Read the model definition and answer for the solid it produces. Units are mm, in the model's axes. Face numbers are marked on the shaded views. A direction names the side the tool comes from. Give positions to 0.01 mm unless a question says otherwise; leave off trailing zeros. Order: outer loops, then holes, each group sorted by start corner. A loop starts at its lowest first (then second) coordinate and runs counter-clockwise, first axis right, second up. Notation, with made-up numbers: (48, 70) - (70, 70) arc R20 cw to (70, 77) - close; hole circle Ø6 at (85.5, 44.25). An arc over 180 degrees is marked (long way). Use a Markdown table: item, result. Add a question column.
1. Which of the six approach directions +Z, -Z, +X, -X, +Y, -Y give full straight-line access (tool end or side, diameter ignored) to the marked faces 4, 5 and 6?
2. A cutting plane is placed at A-A on z = -11. Determine the outline of the cut face in (x, y) (1 decimal).
3. For a pull along X with two mould halves and no side action, classify the marked faces 1, 2 and 3 as released by +X, released by -X, zero draft, split by the parting line, or undercut.
4. Flat-ended cylindrical pins translate along their axes: P1, Ø3, axis at x = 14, z = -22.5, coming from the +Y side; P2, Ø1, axis at x = 20, z = -21, coming from the +Y side; P3, Ø6, axis at x = 3.5, z = -13, coming from the +Y side; P4, Ø3.5, axis at y = 0, z = 0, coming from the +X side. Find the tip coordinate at first contact, or state that the pin passes through.
5. A cutting plane is placed at D-D on x = 16.25. Determine the outline of the cut face in (y, z), and give its area (3 significant figures).
6. Consider L1, parallel to X at y = 1, z = -9 (1 decimal); L2, parallel to Y at x = 26, z = -14.5; L3, parallel to Z at x = 2.5, y = 0. Determine where each line is inside the solid, lowest interval first.
7. A cutting plane is placed at B-B on x = 22.25. Determine the outline of the cut face in (y, z) (1 decimal), and give its area (3 significant figures).
8. A cutting plane is placed at C-C on z = -1.5. Determine the outline of the cut face in (x, y) (1 decimal), and give its area (3 significant figures).
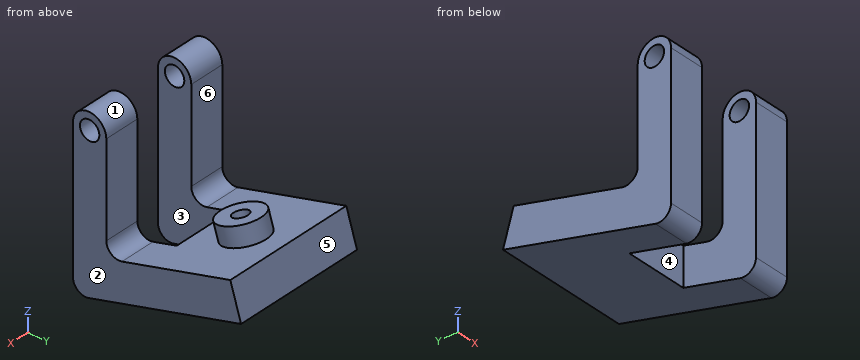
```python
from build123d import *

# Parameters (mm, degrees)
SKETCH1_R               = 2.032
BOSS_EXTRUDE1_DEPTH     = 27.305
FILLET1_R               = 2.54
SKETCH2_W               = 12.7
SKETCH2_H               = 15.24
CUT_EXTRUDE1_DEPTH      = 4.4925
CUT_EXTRUDE1_DEPTH_BACK = 33.127387008
SKETCH3_R               = 4.445
SKETCH3_R_2             = 1.5875
BOSS_EXTRUDE2_DEPTH     = 3.796503


with BuildPart() as part:
    # Sketch1 → Boss-Extrude1 (new body)
    with BuildSketch(Plane(origin=(0, 0, 0), x_dir=(0, 0, -1), z_dir=(1, 0, 0))):
        with BuildLine():
            Line((0, 3.4925), (22.86, 3.4925))
            Line((22.86, 3.4925), (14.913420462, 29.48459049))
            Line((14.913420462, 29.48459049), (22.251950115, 31.728204162))
            Line((22.251950115, 31.728204162), (33.02, -3.4925))
            Line((33.02, -3.4925), (0, -3.4925))
            ThreePointArc((0, -3.4925), (-3.4925, 0), (0, 3.4925))
        make_face()
        Circle(SKETCH1_R, mode=Mode.SUBTRACT)
    extrude(amount=BOSS_EXTRUDE1_DEPTH)

    # Fillet1
    fillet1_edges = [part.edges().sort_by_distance(p)[0] for p in [
        (13.6525, 3.4925, -22.86),
        (13.6525, -3.4925, -33.02),
    ]]
    fillet(fillet1_edges, radius=FILLET1_R)

    # Sketch2 → Cut-Extrude1 (cut, two sides)
    with BuildSketch(Plane.XY) as cut_extrude1_sk:
        with Locations((13.6525, 4.1275)):
            Rectangle(SKETCH2_W, SKETCH2_H)
    extrude(amount=CUT_EXTRUDE1_DEPTH, mode=Mode.SUBTRACT)
    extrude(cut_extrude1_sk.sketch, amount=-CUT_EXTRUDE1_DEPTH_BACK, mode=Mode.SUBTRACT)

    # Sketch3 → Boss-Extrude2 (add)
    with BuildSketch(Plane(origin=(0, 6.690118026, -21.882390062), x_dir=(1, 0, 0), z_dir=(0, -0.292371705, 0.956304756))):
        with Locations((13.6525, 14.562227295)):
            Circle(SKETCH3_R)
        with Locations((13.6525, 14.562227295)):
            Circle(SKETCH3_R_2, mode=Mode.SUBTRACT)
    extrude(amount=BOSS_EXTRUDE2_DEPTH)


solid = part.part
```
Output values:
| question | item | result |
|---|---|---|
| 1 | face 4 | +Z, -Z, -Y |
| 1 | face 5 | +Z, +X, -X, +Y |
| 1 | face 6 | +Z, +X, -X |
| 2 | outline | (0, -3.5) - (7.3, -3.5) - (7.3, 3.5) - (0, 3.5) - close; (20, -3.5) - (27.3, -3.5) - (27.3, 3.5) - (20, 3.5) - close |
| 3 | face 1 | zero draft |
| 3 | face 2 | released by +X |
| 3 | face 3 | undercut |
| 4 | P1 | y = 31.73 |
| 4 | P2 | y = 31.5 |
| 4 | P3 | y = 29.82 |
| 4 | P4 | through |
| 5 | outline | (11.75, -28.36) - (31.73, -22.25) - (29.48, -14.91) - (24.07, -16.57) - (22.96, -12.94) - (16.06, -15.05) - (17.17, -18.68) - (11.75, -20.34) - close |
| 5 | area | 179 mm² |
| 6 | L1 | 0 to 7.3, 20 to 27.3 |
| 6 | L2 | -3.49 to 3.49 |
| 6 | L3 | -31.95 to -2.03, 2.03 to 3.49 |
| 7 | outline | (-3.5, -29.6) arc R2.5 ccw to (-0.2, -32) - (31.7, -22.3) - (29.5, -14.9) - (6.8, -21.9) arc R2.5 cw to (3.5, -19.4) - (3.5, 0) arc R3.5 ccw to (-3.5, 0) - close; hole circle Ø4.1 at (0, 0) |
| 7 | area | 447 mm² |
| 8 | outline | (0, -3.5) - (7.3, -3.5) - (7.3, -1.4) - (0, -1.4) - close; (0, 1.4) - (7.3, 1.4) - (7.3, 3.5) - (0, 3.5) - close; (20, -3.5) - (27.3, -3.5) - (27.3, -1.4) - (20, -1.4) - close; (20, 1.4) - (27.3, 1.4) - (27.3, 3.5) - (20, 3.5) - close |
| 8 | area | 62.0 mm² |
